Here's how the part is built. I have some questions about the finished solid (model axes, mm). Round coordinates to 2 decimals unless told otherwise and drop trailing zeros. Loops run counter-clockwise (first coordinate to the right, second up) from the corner with the lowest first, then second, coordinate; pieces in that order, holes last. Notation, with made-up numbers: (79, 47.25) -> (130, 47.25) arc R13 ccw to (130, 57.25) -> close; hole circle Ø10 at (21.5, -23). An arc over 180 degrees is marked (long way). Use one line per item in the form item = value. Start each with the question number.
Item 1: If I drill on L1, parallel to X at y = -139, z = 99; L2, parallel to Y at x = 102.5, z = 39, over which ranges is the centre line in solid material (lowest first)? Write a range as [from, to].
Item 2: Thinking about a two-plate mould opening in Y: for faces 1 (the face through (9.39, -87.73, 144.33)), 2 (the face through (0, 3, -3)), 3 (the face through (208.45, -42.62, -9.46)), which applies, released by +Y, released by -Y, zero draft, split by the parting line, or undercut?
Item 3: If we section it at A-A (z = 0): Write out the boundary of the cut face in (x, y) (3 decimals).
Item 4: If we section it at D-D (x = 127): Write out the boundary of the cut face in (y, z).
Item 5: I'm going to push flat-ended pins straight in: pin 1 Ø6 at (y, z) = (10, 109.5) entering from +X; pin 2 Ø4 at (x, z) = (332.5, -30) entering from +Y. Where does each tip first touch, or does it pass through?
Item 6: If we section it at C-C (y = -177): Write out the boundary of the cut face in (x, z), then the cut area to 3 significant figures.
```python
from build123d import *

# Parameters (mm, degrees)
F3_D = 25.4


with BuildPart() as f1:
    # F0 (on Front) → F1 (revolve)
    with BuildSketch(Plane.XZ):
        Polygon((0, 203.2), (0, 0), (403.225, 0), (403.225, 43.65625), (19.05, 43.65625), (19.05, 203.2), align=None)
    revolve(axis=Axis((201.6125, 0, 0), (-1, 0, 0)))

    # F3 (through all)
    with Locations(Plane.YZ.offset(19.05)):
        with Locations((0, 180.975), (90.4875, 156.728947), (156.728947, 90.4875), (180.975, 0), (156.728947, -90.4875), (90.4875, -156.728947), (0, -180.975), (-90.4875, -156.728947), (-156.728947, -90.4875), (-180.975, 0), (-156.728947, 90.4875), (-90.4875, 156.728947)):
            Hole(F3_D / 2)


solid = f1.part
```
Values found:
q1.L1 = [0, 19.05]
q1.L2 = [-19.62, 19.62]
q2.face_1 = undercut
q2.face_2 = zero draft
q2.face_3 = split by the parting line
q3.outline = (0, -203.2) -> (19.05, -203.2) -> (19.05, -193.675) -> (0, -193.675) -> close; (0, -168.275) -> (19.05, -168.275) -> (19.05, -43.656) -> (403.225, -43.656) -> (403.225, 43.656) -> (19.05, 43.656) -> (19.05, 168.275) -> (0, 168.275) -> close; (0, 193.675) -> (19.05, 193.675) -> (19.05, 203.2) -> (0, 203.2) -> close
q4.outline = circle Ø87.31 at (0, 0)
q5.pin_1 = 19.05
q5.pin_2 = 33.49
q6.outline = (0, -99.81) -> (19.05, -99.81) -> (19.05, -12.06) -> (0, -12.06) -> close; (0, 12.06) -> (19.05, 12.06) -> (19.05, 99.81) -> (0, 99.81) -> close
q6.area = 3,340 mm2
